```python
from build123d import *

# Parameters (mm, degrees)
BOSS_EXTRUDE1_DEPTH                                 = 7.5
M4_TAPPED_HOLE1_D                                   = 3.3
SKETCH14_R                                          = 5
CUT_EXTRUDE4_DEPTH                                  = 101.124921973
FILLET1_R                                           = 10
CBORE_FOR_M5_HEX_SOCKET_HEAD_CAP_SCREW1_D           = 5.5
CBORE_FOR_M5_HEX_SOCKET_HEAD_CAP_SCREW1_CBORE_D     = 10
CBORE_FOR_M5_HEX_SOCKET_HEAD_CAP_SCREW1_CBORE_DEPTH = 40
CBORE_FOR_M5_HEX_SOCKET_HEAD_CAP_SCREW2_D           = 5.5
CBORE_FOR_M5_HEX_SOCKET_HEAD_CAP_SCREW2_CBORE_D     = 10
CBORE_FOR_M5_HEX_SOCKET_HEAD_CAP_SCREW2_CBORE_DEPTH = 40
F_5_0_5_DIAMETER_HOLE1_D                            = 5


with BuildPart() as part:
    # Sketch1 → Boss-Extrude1 (new, symmetric)
    with BuildSketch(Plane(origin=(0, 0, 0), x_dir=(1, 0, 0), z_dir=(0, 1, 0))):
        Polygon((-20, 20), (-20, -20), (20, -20), (20, -30), (-40, -70), (-70, -70), (-70, -30), (-30, 20), align=None)
    extrude(amount=BOSS_EXTRUDE1_DEPTH, both=True)

    # M4 Tapped Hole1 (through all)
    with Locations(Plane(origin=(0, 7.5, 0), x_dir=(1, 0, 0), z_dir=(0, 1, 0))):
        with Locations((-55, -27.5), (-55, -64)):
            Hole(M4_TAPPED_HOLE1_D / 2)

    # Sketch14 → Cut-Extrude4 (cut, through all)
    with BuildSketch(Plane(origin=(0, 7.5, 0), x_dir=(1, 0, 0), z_dir=(0, 1, 0))):
        with Locations(Location((-55, -45.75, 0), (0, 0, 270))):
            Circle(SKETCH14_R)
    extrude(amount=-CUT_EXTRUDE4_DEPTH, mode=Mode.SUBTRACT)

    # Fillet1
    fillet1_edges = [part.edges().sort_by_distance(p)[0] for p in [
        (-40, 0, 70),
        (-70, 0, 70),
        (-70, 0, 30),
    ]]
    fillet(fillet1_edges, radius=FILLET1_R)

    # CBORE for M5 Hex Socket Head Cap Screw1 (through all)
    with Locations(Plane.XY.offset(70)):
        with Locations((10, 0), (-10, 0)):
            CounterBoreHole(CBORE_FOR_M5_HEX_SOCKET_HEAD_CAP_SCREW1_D / 2, CBORE_FOR_M5_HEX_SOCKET_HEAD_CAP_SCREW1_CBORE_D / 2, CBORE_FOR_M5_HEX_SOCKET_HEAD_CAP_SCREW1_CBORE_DEPTH)

    # CBORE for M5 Hex Socket Head Cap Screw2 (through all)
    with Locations(Plane.ZY.offset(70)):
        with Locations((10, 0), (-10, 0)):
            CounterBoreHole(CBORE_FOR_M5_HEX_SOCKET_HEAD_CAP_SCREW2_D / 2, CBORE_FOR_M5_HEX_SOCKET_HEAD_CAP_SCREW2_CBORE_D / 2, CBORE_FOR_M5_HEX_SOCKET_HEAD_CAP_SCREW2_CBORE_DEPTH)

    # 5.0 _5_ Diameter Hole1 (through all)
    with Locations(Plane(origin=(0, 7.5, 0), x_dir=(1, 0, 0), z_dir=(0, 1, 0))):
        with Locations((-20, -20)):
            Hole(F_5_0_5_DIAMETER_HOLE1_D / 2)


solid = part.part
```
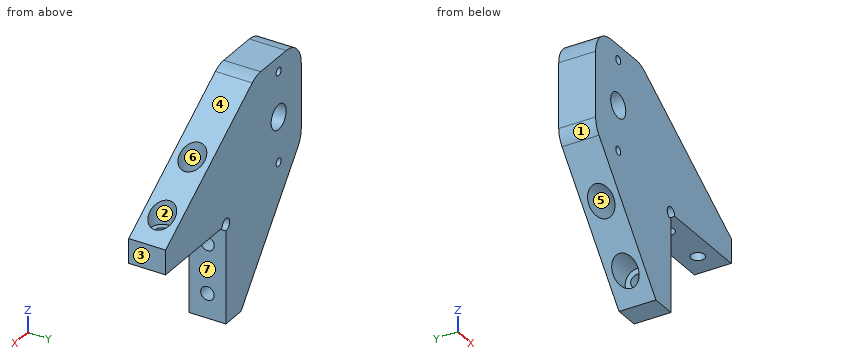
Read the model definition and answer for the solid it produces. Units are mm, in the model's axes. Face numbers are marked on the shaded views. A direction names the side the tool comes from. Coordinates: 2 decimals unless noted, no trailing zeros. Loops run counter-clockwise (first coordinate to the right, second up) from the corner with the lowest first, then second, coordinate; pieces in that order, holes last. Notation, with made-up numbers: (22.5, 40.25) - (49.5, 40.25) arc R29 cw to (49.5, 65.25) - close; hole circle Ø6 at (3.25, 51). An arc over 180 degrees is marked (long way). Answer in a Markdown table with one row per item.
1. Find section D-D, the plane x = 10. Write down the section's boundary in (y, z), then the cut area to 3 significant figures.
Conclusion:
| item | result |
|---|---|
| outline | (-7.5, 20) - (-2.75, 20) - (-2.75, 30) - (-5, 30) - (-5, 36.67) - (-7.5, 36.67) - close; (2.75, 20) - (7.5, 20) - (7.5, 36.67) - (5, 36.67) - (5, 30) - (2.75, 30) - close |
| area | 128 mm² |
2. Determine the mould class of the marked faces 1, 2 and 3 for opening direction X: +X half, -X half, draft (parallel to the pull), parting line (faces both ways), or undercut.
Conclusion:
| item | result |
|---|---|
| face 1 | -X half |
| face 2 | undercut |
| face 3 | +X half |
3. Find section B-B, the plane z = -10. Write down the section's boundary in (x, y), then the cut area to 3 significant figures.
Conclusion:
| item | result |
|---|---|
| outline | (-38, -7.5) - (-20, -7.5) - (-20, -2.75) - (-30, -2.75) - (-30, -5) - (-38, -5) - close; (-38, 5) - (-30, 5) - (-30, 2.75) - (-20, 2.75) - (-20, 7.5) - (-38, 7.5) - close |
| area | 135 mm² |
4. Straight lines are drawn through the part: line 1 (Y direction, x = -10.5, z = 37); line 2 (X direction, y = 0, z = 39.75); line 3 (Y direction, x = -10, z = 27). For each, find the intervals that lie inside material, in ascending order.
Conclusion:
| item | result |
|---|---|
| line 1 | y = -7.5 to -4.97, 4.97 to 7.5 |
| line 2 | x = -70 to -15, -5 to 5 |
| line 3 | y = -7.5 to -2.75, 2.75 to 7.5 |
5. Find section A-A, the plane x = -34. Write down the section's boundary in (y, z), then the cut area to 3 significant figures.
Conclusion:
| item | result |
|---|---|
| outline | (-7.5, -15) - (7.5, -15) - (7.5, 66) - (-7.5, 66) - close; hole circle Ø10 at (0, -10); hole circle Ø10 at (0, 10) |
| area | 1,060 mm² |
6. Which of the six approach directions +Z, -Z, +X, -X, +Y, -Y give full straight-line access (tool end or side, diameter ignored) to the marked faces 4, 5, 6 and 7?
Conclusion:
| item | result |
|---|---|
| face 4 | +Z, +X, +Y, -Y |
| face 5 | -X |
| face 6 | +Z |
| face 7 | -Z, +X, +Y, -Y |
7. Find section C-C, the plane x = -55. Write down the section's boundary in (y, z), then the cut area to 3 significant figures.
Conclusion:
| item | result |
|---|---|
| outline | (-7.5, 11.25) - (-4.84, 11.25) arc R5 cw to (4.84, 11.25) - (7.5, 11.25) - (7.5, 25.85) - (-7.5, 25.85) - close; (-7.5, 29.15) - (7.5, 29.15) - (7.5, 40.75) - (-7.5, 40.75) - close; (-7.5, 50.75) - (7.5, 50.75) - (7.5, 62.35) - (-7.5, 62.35) - close; (-7.5, 65.65) - (7.5, 65.65) - (7.5, 70) - (-7.5, 70) - close |
| area | 605 mm² |
8. Given pin 1 (7.5 mm diameter, centred on y = -2, z = 3.5, fed in from +X); pin 2 (8 mm diameter, centred on y = -0.5, z = 17.5, fed in from -X); pin 3 (8 mm diameter, centred on y = -1.5, z = -11, fed in from -X), each flat-ended and moving along its own axis, determine where each tip first touches the part or whether it passes through.
Conclusion:
| item | result |
|---|---|
| pin 1 | stops at x = -20 |
| pin 2 | stops at x = -63.2 |
| pin 3 | stops at x = -38.93 |
